Here's how the part is built. I have some questions about the finished solid (model axes, mm). Face numbers are marked on the shaded views. A direction names the side the tool comes from. Round coordinates to 2 decimals unless told otherwise and drop trailing zeros. Loops run counter-clockwise (first coordinate to the right, second up) from the corner with the lowest first, then second, coordinate; pieces in that order, holes last. Notation, with made-up numbers: (58.5, 76.25) - (77.5, 76.25) arc R16 ccw to (77.5, 80.25) - close; hole circle Ø9 at (26, -27). An arc over 180 degrees is marked (long way). Answer as a JSON object with one key per item and string values. Group by question number.
1) I want a section at A-A, the plane y = 12.7. Please give me the cut outline in (x, z) (3 decimals).
2) Will these pins go through, and if not, where does the flat tip stop? P1, Ø3, axis at x = -68, y = 5.5, coming from the -Z side; P2, Ø3, axis at x = -9.5, y = 6.5, coming from the -Z side; P3, Ø11.5, axis at x = -26, y = 17.5, coming from the -Z side (3 decimals).
3) If I drill on line 1 along Z through (x, y) = (-82.5, 19.25) (3 decimals); line 2 along Y through (x, z) = (-19.5, -12) (3 decimals); line 3 along Z through (x, y) = (-68.5, 4.75), over which ranges is the centre line in solid material (lowest first)? Write a range as [from, to].
4) I want a section at D-D, the plane z = -20.75. Please give me the cut outline in (x, y) (3 decimals), then the cut area to 3 significant figures.
5) Which directions (+Z, -Z, +X, -X, +Y, -Y) give clear straight access to the entire face, cutting with the end or side of a thin tool? Please do the marked faces 1 and 2.
from build123d import *

# Parameters (mm, degrees)
MIEMBRO_ESTRUCTURAL1_DEPTH    = 106
TALADRO_DE_MARGEN_PARA_1_41_D = 6.7564


with BuildPart() as part:
    # Sketch12 → Miembro estructural1 (new body)
    with BuildSketch(Plane(origin=(-95.224809186, 0, 0), x_dir=(0, 0, -1), z_dir=(1, 0, 0))):
        with BuildLine():
            Line((0, 0), (0, 25.4))
            Line((0, 25.4), (0.00508, 25.4))
            ThreePointArc((0.00508, 25.4), (2.246551928, 24.471551928), (3.175, 22.23008))
            Line((3.175, 22.23008), (3.175, 7.9375))
            ThreePointArc((3.175, 7.9375), (4.569903955, 4.569903955), (7.9375, 3.175))
            Line((7.9375, 3.175), (22.23008, 3.175))
            ThreePointArc((22.23008, 3.175), (24.471551928, 2.246551928), (25.4, 0.00508))
            Line((25.4, 0.00508), (25.4, 0))
            Line((25.4, 0), (0, 0))
        make_face()
    extrude(amount=MIEMBRO_ESTRUCTURAL1_DEPTH)

    # Taladro de margen para 1/41 (through all)
    with Locations(Plane.XY):
        with Locations((-35.224809186, 12.7), (-75.224809186, 12.7)):
            Hole(TALADRO_DE_MARGEN_PARA_1_41_D / 2)


solid = part.part
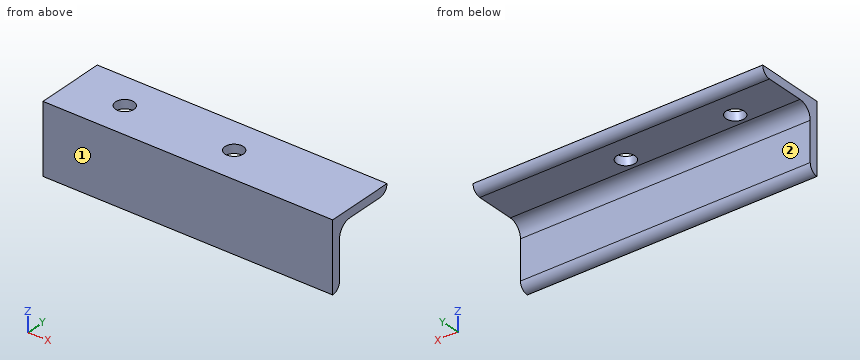
Outcome:
{
 "1": {"outline": "(-95.225, -3.175) - (-78.603, -3.175) - (-78.603, 0) - (-95.225, 0) - close; (-71.847, -3.175) - (-38.603, -3.175) - (-38.603, 0) - (-71.847, 0) - close; (-31.847, -3.175) - (10.775, -3.175) - (10.775, 0) - (-31.847, 0) - close"},
 "2": {"P1": "z = -5.26", "P2": "z = -4.19", "P3": "z = -3.175"},
 "3": {"line 1": "[-3.175, 0]", "line 2": "[0, 3.175]", "line 3": "[-4.4, 0]"},
 "4": {"outline": "(-95.225, 0) - (10.775, 0) - (10.775, 3.175) - (-95.225, 3.175) - close", "area": "337 mm^2"},
 "5": {"face 1": "+Z, -Z, +X, -X, -Y", "face 2": "-Z, +X, -X, +Y"}
}
